from build123d import *

# Parameters (mm, degrees)
ESTRUSIONE_ESTRUSIONE1_DEPTH             = 2
RACCORDO1_R                              = 1
RACCORDO2_R                              = 0.5
ESTRUSIONE_ESTRUSIONE2_DEPTH             = 2.5
ESTRUSIONE_ESTRUSIONE2_DEPTH_BACK        = 1.5
SCHIZZO2_R                               = 3
ESTRUSIONE_ESTRUSIONE3_REACH             = 20.507
ESTRUSIONE_ESTRUSIONE3_DIRECTION_2_REACH = 20.507
ESTRUSIONE_ESTRUSIONE4_DEPTH             = 3
RACCORDO3_R                              = 0.5
SCHIZZO5_R                               = 1.5
TAGLIO_ESTRUSIONE1_DEPTH                 = 21.528432045
ESTRUSIONE_ESTRUSIONE5_DEPTH             = 0.1


with BuildPart() as part:
    # Schizzo1 → Estrusione-Estrusione1 (new body)
    with BuildSketch(Plane.XY):
        Polygon((-16.707106781, 0.792893219), (-10.707106781, 0.792893219), (-10, 1.5), (0, 1.5), (0, 3.5), (15, 3.5), (15, 0), (15, -1.154985921), (9.361844275, -3.207106781), (-11.638155725, -3.207106781), (-11.638155725, -1.207106781), (-16.707106781, -1.207106781), align=None)
    extrude(amount=ESTRUSIONE_ESTRUSIONE1_DEPTH)

    # Raccordo1
    raccordo1_edges = [part.edges().sort_by_distance(p)[0] for p in [
        (-11.638155725, -3.207106781, 1),
    ]]
    fillet(raccordo1_edges, radius=RACCORDO1_R)

    # Raccordo2
    raccordo2_edges = [part.edges().sort_by_distance(p)[0] for p in [
        (-11.638155725, -1.207106781, 1),
    ]]
    fillet(raccordo2_edges, radius=RACCORDO2_R)

    # Schizzo2 → Estrusione-Estrusione2 (add, two sides: drawn at the far end of the back side and taken through both)
    with BuildSketch(Plane.XY.offset(-ESTRUSIONE_ESTRUSIONE2_DEPTH_BACK)):
        with Locations((15, 0.5)):
            Circle(SCHIZZO2_R)
    extrude(amount=ESTRUSIONE_ESTRUSIONE2_DEPTH + ESTRUSIONE_ESTRUSIONE2_DEPTH_BACK)

    # Estrusione-Estrusione3: up to this face of the body (flat: up to its plane)
    estrusione_estrusione3_end = Plane(part.part.faces().sort_by_distance((0.378494116, -0.204899382, 2))[0])
    # Schizzo3 → Estrusione-Estrusione3 (add, up to the picked face)
    with BuildSketch(Plane.XY, mode=Mode.PRIVATE) as estrusione_estrusione3_sk1:
        with BuildLine():
            Line((18.828427125, 1.5), (17.828427125, 1.5))
            ThreePointArc((17.828427125, 1.5), (18, 0.5), (17.828427125, -0.5))
            Line((17.828427125, -0.5), (18.828427125, -0.5))
            ThreePointArc((18.828427125, -0.5), (19.828427125, 0.5), (18.828427125, 1.5))
        make_face()
    estrusione_estrusione3_tool1 = split(extrude(estrusione_estrusione3_sk1.sketch, amount=ESTRUSIONE_ESTRUSIONE3_REACH, mode=Mode.PRIVATE), bisect_by=estrusione_estrusione3_end, keep=Keep.BOTH, mode=Mode.PRIVATE)
    add(estrusione_estrusione3_tool1.solids().sort_by(Axis((18.792788, 0.5, 0), (0, 0, 1)))[0])

    # Estrusione-Estrusione3 direction 2: up to this face of the body (flat: up to its plane)
    estrusione_estrusione3_direction_2_end = Plane(part.part.faces().sort_by_distance((15, 0.5, -1.5))[0])
    # Schizzo3 → Estrusione-Estrusione3 direction 2 (add, up to the picked face)
    with BuildSketch(Plane.XY, mode=Mode.PRIVATE) as estrusione_estrusione3_direction_2_sk1:
        with BuildLine():
            Line((18.828427125, 1.5), (17.828427125, 1.5))
            ThreePointArc((17.828427125, 1.5), (18, 0.5), (17.828427125, -0.5))
            Line((17.828427125, -0.5), (18.828427125, -0.5))
            ThreePointArc((18.828427125, -0.5), (19.828427125, 0.5), (18.828427125, 1.5))
        make_face()
    estrusione_estrusione3_direction_2_tool1 = split(extrude(estrusione_estrusione3_direction_2_sk1.sketch, amount=-ESTRUSIONE_ESTRUSIONE3_DIRECTION_2_REACH, mode=Mode.PRIVATE), bisect_by=estrusione_estrusione3_direction_2_end, keep=Keep.BOTH, mode=Mode.PRIVATE)
    add(estrusione_estrusione3_direction_2_tool1.solids().sort_by(Axis((18.792788, 0.5, 0), (0, 0, -1)))[0])

    # Schizzo4 → Estrusione-Estrusione4 (add)
    with BuildSketch(Plane.ZY.offset(16.707106781)):
        Polygon((2, -1.207106781), (3.5, -1.207106781), (3.5, -3.307106781), (4, -3.307106781), (4, 0.192893219), (2, 0.192893219), align=None)
    extrude(amount=-ESTRUSIONE_ESTRUSIONE4_DEPTH)

    # Raccordo3
    raccordo3_edges = [part.edges().sort_by_distance(p)[0] for p in [
        (-15.207106781, 0.192893219, 4),
        (-13.707106781, -1.557106781, 4),
        (-15.207106781, -3.307106781, 4),
        (-16.707106781, -1.557106781, 4),
    ]]
    fillet(raccordo3_edges, radius=RACCORDO3_R - 0.0001)  # a hair under: the kernel refuses the full size

    # Schizzo5 → Taglio-Estrusione1 (cut, through all)
    with BuildSketch(Plane.XY.offset(2.5)):
        with Locations((15, 0.5)):
            Circle(SCHIZZO5_R)
    extrude(amount=-TAGLIO_ESTRUSIONE1_DEPTH, mode=Mode.SUBTRACT)


with BuildPart() as body_2:
    # Specchia2: mirrored copy
    add(part.part.mirror(Plane.ZX))

    # Schizzo6 → Estrusione-Estrusione5 (add)
    with BuildSketch(Plane.XY.offset(2)):
        Polygon((10.5, 0.758388832), (10.5, 0.444286268), (7.358974359, 0.444286268), (7.358974359, -0.901867578), (7, -0.901867578), (7, 0.758388832), align=None)
    extrude(amount=ESTRUSIONE_ESTRUSIONE5_DEPTH)


solid = body_2.part
Check sheet for the modelled part. Datum: model origin and axes. Units: mm. A direction names the side the tool comes from. Coordinates: 2 decimals unless noted, no trailing zeros. Write each loop counter-clockwise with the first axis right and the second up, starting at its lowest first coordinate (ties: lowest second). Pieces come first, ordered by that corner, then holes.
Item 1: Scan lines: probe 1 along X at (y, z) = (-0.5, 0.5); probe 2 along X at (y, z) = (-0.5, -0.35); probe 3 along Z at (x, y) = (-3.5, 1.75). Record each from-to range of solid material in increasing order.
Numbers:
probe 1: x = -16.71 to 13.5, 16.5 to 19.83
probe 2: x = 12 to 13.5, 16.5 to 19.83
probe 3: z = 0 to 2
Item 2: Mould release check, pull along Y, two halves, no side actions. Record for faces 1 (the face through (8.2, 0.6, 2.1)), 2 (the face through (13.5, -0.57, 0.53)), 3 (the face through (11.3, 2.5, 1)): released by +Y, released by -Y, zero draft, split by the parting line, or undercut.
Numbers:
face 1: zero draft
face 2: undercut
face 3: released by +Y
Item 3: Cross-section at B-B on x = 14. Record the boundary of the cut face in (y, z), then the cut area to 3 significant figures.
Numbers:
outline: (-3.5, 0) - (-3.33, 0) - (-3.33, -1.5) - (-1.62, -1.5) - (-1.62, 2.5) - (-3.33, 2.5) - (-3.33, 2) - (-3.5, 2) - close; (0.62, -1.5) - (2.33, -1.5) - (2.33, 2.5) - (0.62, 2.5) - close
area: 14.0 mm2
Item 4: Cross-section at D-D on z = 3.1. Record the boundary of the cut face in (x, y), then the cut area to 3 significant figures.
Numbers:
outline: (-16.71, -0.19) - (-13.71, -0.19) - (-13.71, 1.21) - (-16.71, 1.21) - close
area: 4.20 mm2
Item 5: Access from +Z, -Z, +X, -X, +Y, -Y to the whole of each face (thin tool, end or side, straight path). Record for faces 4 (the face through (-15, -0.193, 3)), 5 (the face through (16, -2, 2.5)), 6 (the face through (-5, -1.5, 1)), 7 (the face through (-13.707, 1, 3)).
Numbers:
face 4: +Z, -X, -Y
face 5: +Z, +X, +Y, -Y
face 6: +Z, -Z, -X, -Y
face 7: +Z, +Y, -Y
Item 6: Depth check by flat-ended pin: pin 1 Ø3.5 at (x, y) = (-4.5, -1) entering from -Z; pin 2 Ø2 at (x, z) = (11.5, 0) entering from +Y; pin 3 Ø1.8 at (x, y) = (14.5, -1) entering from +Z. Enter the tip coordinate at first touch or a pass-through.
Numbers:
pin 1: stops at z = 0
pin 2: stops at y = 2.79
pin 3: stops at z = 2.5
Item 7: Cross-section at C-C on z = -0.9. Record the boundary of the cut face in (x, y).
Numbers:
outline: (17.83, -1.5) - (18.83, -1.5) arc R1 ccw to (18.83, 0.5) - (17.83, 0.5) arc R3 ccw (long way) to start; hole circle Ø3 at (15, -0.5)
Item 8: Cross-section at A-A on z = 0.8. Record the boundary of the cut face in (x, y), then the cut area to 3 significant figures.
Numbers:
outline: (-16.71, -0.79) - (-10.71, -0.79) - (-10, -1.5) - (0, -1.5) - (0, -3.5) - (15, -3.5) arc R3 ccw to (17.83, -1.5) - (18.83, -1.5) arc R1 ccw to (18.83, 0.5) - (17.83, 0.5) arc R3 ccw to (13.12, 1.84) - (9.36, 3.21) - (-10.64, 3.21) arc R1 ccw to (-11.64, 2.21) - (-11.64, 1.71) arc R0.5 cw to (-12.14, 1.21) - (-16.71, 1.21) - close; hole circle Ø3 at (15, -0.5)
area: 171 mm2
